from build123d import *

# Parameters (mm, degrees)
BOSS_EXTRUDE1_DEPTH  = 75
SKETCH2_R            = 7.5
SKETCH2_R_2          = 5
SKETCH2_W            = 75
SKETCH2_H            = 23.9
CUT_EXTRUDE1_DEPTH   = 75
M6_CLEARANCE_HOLE1_D = 6.4


with BuildPart() as part:
    # Sketch1 → Boss-Extrude1 (new body)
    with BuildSketch(Plane(origin=(0, 0, 0), x_dir=(0, 0, -1), z_dir=(1, 0, 0))):
        with BuildLine():
            Line((0, 0), (0, 88.9))
            Line((0, 88.9), (6.35, 88.9))
            Line((6.35, 88.9), (6.35, 15.875))
            ThreePointArc((6.35, 15.875), (9.139807909, 9.139807909), (15.875, 6.35))
            Line((15.875, 6.35), (40, 6.35))
            Line((40, 6.35), (40, 0))
            Line((40, 0), (0, 0))
        make_face()
    extrude(amount=BOSS_EXTRUDE1_DEPTH)

    # Sketch2 → Cut-Extrude1 (cut)
    with BuildSketch(Plane(origin=(0, 0, 0), x_dir=(-1, 0, 0), z_dir=(0, 0, -1))):
        with Locations((-30, 50.875)):
            Circle(SKETCH2_R)
        with Locations((-45, 50.875)):
            Circle(SKETCH2_R_2)
        with Locations((-37.5, 76.95)):
            Rectangle(SKETCH2_W, SKETCH2_H)
    extrude(amount=CUT_EXTRUDE1_DEPTH, mode=Mode.SUBTRACT)

    # M6 Clearance Hole1 (through all)
    with Locations(Plane(origin=(12.5, 0, -25), x_dir=(0, 0, -1), z_dir=(0, -1, 0))):
        with Locations((0, 0), (0, 50)):
            Hole(M6_CLEARANCE_HOLE1_D / 2)


solid = part.part
Model file for the job. Use its own axes, mm. A direction names the side the tool comes from. Coordinates: 2 decimals unless noted, no trailing zeros. Order: outer loops, then holes, each group sorted by start corner. A loop starts at its lowest first (then second) coordinate and runs counter-clockwise, first axis right, second up. Notation, with made-up numbers: (71.25, -3.75) -> (119.25, -3.75) arc R30 ccw to (119.25, 30.25) -> close; hole circle Ø9 at (76, 82.25). An arc over 180 degrees is marked (long way). Return JSON: item names as keys, results as strings. Group by question number.
Item 1: Saw through at B-B on x = 62.5. Write the cut outline in (y, z) (3 decimals).
Item 2: Saw through at D-D on x = 45. Write the cut outline in (y, z) (3 decimals), then the cut area to 3 significant figures.
Item 3: Saw through at C-C on y = 55. Write the cut outline in (x, z).
Item 4: Pull direction X, two halves, no side cores. Call faces 3 (the cylindrical face through (36.98, 9.21, -9.07)), 4 (the cylindrical face through (12.6, 3.2, -28.2)), 5 (the cylindrical face through (31.626, 43.553, -3.131)), 6 (the flat face through (75, 23, -5)): pulls with the +X half, pulls with the -X half, needs draft (parallel to the pull), parting line crosses it, or undercut.
Item 5: Wall check: line 1 along X through (y, z) = (4, -25); line 2 along Y through (x, z) = (45, -5) (3 decimals); line 3 along Z through (x, y) = (16, 19.5). Give the ranges that are in metal, low to high. Write a range as [from, to].
Item 6: Saw through at A-A on z = -25. Write the cut outline in (x, y).
Item 7: Tool access for faces 1 (the flat face through (37, 41, -6.35)), 2 (the flat face through (37, 32, 0)): list every direction of +Z, -Z, +X, -X, +Y, -Y with a clear straight run to the whole face (end or side of a thin tool).
Item 8: Flat gauge pins, fed straight in: P1, Ø13, axis at x = 45, y = 50.875, coming from the -Z side; P2, Ø3, axis at x = 9.5, z = -27.5, coming from the +Y side. Where does each tip first touch, or does it go through?
Values found:
{
 "1": {"outline": "(0, -40) -> (6.35, -40) -> (6.35, -28.2) -> (0, -28.2) -> close; (0, -21.8) -> (6.35, -21.8) -> (6.35, -15.875) arc R9.525 cw to (15.875, -6.35) -> (65, -6.35) -> (65, 0) -> (0, 0) -> close"},
 "2": {"outline": "(0, -40) -> (6.35, -40) -> (6.35, -15.875) arc R9.525 cw to (15.875, -6.35) -> (45.875, -6.35) -> (45.875, 0) -> (0, 0) -> close; (55.875, -6.35) -> (65, -6.35) -> (65, 0) -> (55.875, 0) -> close", "area": "582 mm2"},
 "3": {"outline": "(0, -6.35) -> (23.74, -6.35) -> (23.74, 0) -> (0, 0) -> close; (36.26, -6.35) -> (42.17, -6.35) -> (42.17, 0) -> (36.26, 0) -> close; (47.83, -6.35) -> (75, -6.35) -> (75, 0) -> (47.83, 0) -> close"},
 "4": {"face 3": "needs draft", "face 4": "undercut", "face 5": "undercut", "face 6": "pulls with the +X half"},
 "5": {"line 1": "x = [0, 9.3], [15.7, 59.3], [65.7, 75]", "line 2": "y = [0, 45.875], [55.875, 65]", "line 3": "z = [-6.35, 0]"},
 "6": {"outline": "(0, 0) -> (9.3, 0) -> (9.3, 6.35) -> (0, 6.35) -> close; (15.7, 0) -> (59.3, 0) -> (59.3, 6.35) -> (15.7, 6.35) -> close; (65.7, 0) -> (75, 0) -> (75, 6.35) -> (65.7, 6.35) -> close"},
 "7": {"face 1": "-Z, +X, -X, +Y", "face 2": "+Z, +X, -X, +Y, -Y"},
 "8": {"P1": "stops at z = -6.35", "P2": "stops at y = 6.35"}
}
